The listing builds one solid part. Answer for the finished solid, in the listing's coordinates (mm). Round coordinates to 2 decimals unless told otherwise and drop trailing zeros. Write each loop counter-clockwise with the first axis right and the second up, starting at its lowest first coordinate (ties: lowest second). Pieces come first, ordered by that corner, then holes. Notation, with made-up numbers: (-16.5, -7.75) - (-9.5, -7.75) arc R12 ccw to (-9.5, 6.25) - close; hole circle Ø3 at (20.25, -12.75). An arc over 180 degrees is marked (long way). Use a Markdown table: item, result. Add a question column.
1) A cutting plane is placed at B-B (z = -87.22). Give the vertices of the cut face in (x, y).
2) A cutting plane is placed at C-C (y = 0.95). Give the vertices of the cut face in (x, z) (3 decimals), then the cut area to 3 significant figures.
3) A cutting plane is placed at A-A (x = 104.18). Give the vertices of the cut face in (y, z) (3 decimals).
4) Find the intervals of material crossed by probe 1 along X at (y, z) = (1.25, -131.5); probe 2 along X at (y, z) = (2.2, -87.22); probe 3 along Z at (x, y) = (18, 1.9), in increasing order. Write a range as from..to.
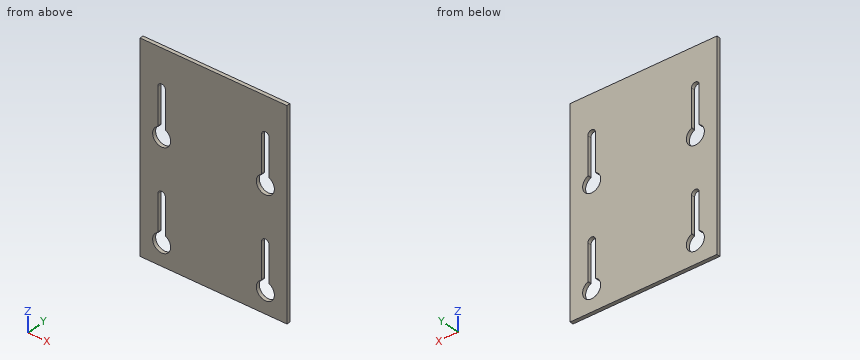
```python
from build123d import *

# Parameters (mm, degrees)
SKETCH3_W           = 122.1
SKETCH3_H           = 197.8
BOSS_EXTRUDE2_DEPTH = 3
SKETCH4_R           = 7.5
CUT_EXTRUDE2_DEPTH  = 3
SKETCH5_W           = 185.639017853
SKETCH5_H           = 93.814581834
CUT_EXTRUDE3_DEPTH  = 12
SKETCH7_W           = 181.97184254
SKETCH7_H           = 161.609726855
CUT_EXTRUDE4_DEPTH  = 19


with BuildPart() as part:
    # Sketch3 → Boss-Extrude2 (new body)
    with BuildSketch(Plane(origin=(0, 0, 0), x_dir=(1, 0, 0), z_dir=(0, 1, 0))):
        with Locations((61.05, 98.9)):
            Rectangle(SKETCH3_W, SKETCH3_H)
    extrude(amount=BOSS_EXTRUDE2_DEPTH)

    # Sketch4 → Cut-Extrude2 (cut)
    with BuildSketch(Plane(origin=(0, 3, 0), x_dir=(1, 0, 0), z_dir=(0, 1, 0))):
        with Locations((17.92, 168.12)):
            Circle(SKETCH4_R)
        with Locations((17.92, 87.22)):
            Circle(SKETCH4_R)
        with Locations((104.18, 87.22)):
            Circle(SKETCH4_R)
        with Locations((104.18, 168.12)):
            Circle(SKETCH4_R)
        with BuildLine():
            Line((21.08772899, 160.62), (21.08772899, 131.62))
            ThreePointArc((21.08772899, 131.62), (17.92, 128.45227101), (14.75227101, 131.62))
            Line((14.75227101, 131.62), (14.75227101, 160.62))
            ThreePointArc((14.75227101, 160.62), (17.92, 163.78772899), (21.08772899, 160.62))
        make_face()
        with BuildLine():
            Line((21.085, 79.72), (21.085, 49.72))
            ThreePointArc((21.085, 49.72), (17.92, 46.555), (14.755, 49.72))
            Line((14.755, 49.72), (14.755, 79.72))
            ThreePointArc((14.755, 79.72), (17.92, 82.885), (21.085, 79.72))
        make_face()
        with BuildLine():
            Line((101.015, 79.72), (101.015, 49.72))
            ThreePointArc((101.015, 49.72), (104.18, 46.555), (107.345, 49.72))
            Line((107.345, 49.72), (107.345, 79.72))
            ThreePointArc((107.345, 79.72), (104.18, 82.885), (101.015, 79.72))
        make_face()
        with BuildLine():
            Line((101.01227101, 160.62), (101.01227101, 131.62))
            ThreePointArc((101.01227101, 131.62), (104.18, 128.45227101), (107.34772899, 131.62))
            Line((107.34772899, 131.62), (107.34772899, 160.62))
            ThreePointArc((107.34772899, 160.62), (104.18, 163.78772899), (101.01227101, 160.62))
        make_face()
    extrude(amount=-CUT_EXTRUDE2_DEPTH, mode=Mode.SUBTRACT)

    # Sketch5 → Cut-Extrude3 (cut)
    with BuildSketch(Plane(origin=(0, 0, -197.8), x_dir=(-1, 0, 0), z_dir=(0, 0, -1))):
        with Locations((-62.393879106, -6.143731482)):
            Rectangle(SKETCH5_W, SKETCH5_H)
    extrude(amount=-CUT_EXTRUDE3_DEPTH, mode=Mode.SUBTRACT)

    # Sketch7 → Cut-Extrude4 (cut)
    with BuildSketch(Plane.XY):
        with Locations((66.543858185, 9.384028943)):
            Rectangle(SKETCH7_W, SKETCH7_H)
    extrude(amount=-CUT_EXTRUDE4_DEPTH, mode=Mode.SUBTRACT)


solid = part.part
```
Entries:
| question | item | result |
|---|---|---|
| 1 | outline | (0, 0) - (10.42, 0) - (10.42, 3) - (0, 3) - close; (25.42, 0) - (96.68, 0) - (96.68, 3) - (25.42, 3) - close; (111.68, 0) - (122.1, 0) - (122.1, 3) - (111.68, 3) - close |
| 2 | outline | (0, -185.8) - (122.1, -185.8) - (122.1, -19) - (0, -19) - close; hole (14.752, -160.62) arc R3.168 ccw to (14.824, -161.289) arc R7.5 ccw (long way) to (21.016, -161.289) arc R3.168 ccw to (21.088, -160.62) - (21.088, -131.62) arc R3.168 ccw to (14.752, -131.62) - close; hole (14.755, -79.72) arc R3.165 ccw to (14.826, -80.388) arc R7.5 ccw (long way) to (21.014, -80.388) arc R3.165 ccw to (21.085, -79.72) - (21.085, -49.72) arc R3.165 ccw to (14.755, -49.72) - close; hole (101.012, -160.62) arc R3.168 ccw to (101.084, -161.289) arc R7.5 ccw (long way) to (107.276, -161.289) arc R3.168 ccw to (107.348, -160.62) - (107.348, -131.62) arc R3.168 ccw to (101.012, -131.62) - close; hole (101.015, -79.72) arc R3.165 ccw to (101.086, -80.388) arc R7.5 ccw (long way) to (107.274, -80.388) arc R3.165 ccw to (107.345, -79.72) - (107.345, -49.72) arc R3.165 ccw to (101.015, -49.72) - close |
| 2 | area | 18,800 mm² |
| 3 | outline | (0, -185.8) - (3, -185.8) - (3, -175.62) - (0, -175.62) - close; (0, -128.452) - (3, -128.452) - (3, -94.72) - (0, -94.72) - close; (0, -46.555) - (3, -46.555) - (3, -19) - (0, -19) - close |
| 4 | probe 1 | x = 0..14.75, 21.09..101.01, 107.35..122.1 |
| 4 | probe 2 | x = 0..10.42, 25.42..96.68, 111.68..122.1 |
| 4 | probe 3 | z = -185.8..-175.62, -128.45..-94.72, -46.56..-19 |
